Read the model definition and answer for the solid it produces. Units are mm, in the model's axes. Coordinates: 2 decimals unless noted, no trailing zeros. Loops run counter-clockwise (first coordinate to the right, second up) from the corner with the lowest first, then second, coordinate; pieces in that order, holes last. Notation, with made-up numbers: (83, 8) -> (95, 8) arc R14 cw to (95, 12) -> close; hole circle Ø7 at (33, -29.5). An arc over 180 degrees is marked (long way). Answer as a JSON object with one key per item and string values. Group by question number.
Q1. The part is cut by section D-D on x = 9.63. Write down the section's boundary in (y, z) (3 decimals), and give its area (3 significant figures).
Q2. The part is cut by section A-A on x = -12.5. Write down the section's boundary in (y, z) (3 decimals), and give its area (3 significant figures).
Q3. Straight lines are drawn through the part: line 1 along X through (y, z) = (0.7, 9.5); line 2 along X through (y, z) = (0.5, 8.5); line 3 along X through (y, z) = (1.45, -0.5). For each, find the intervals that lie inside material, in ascending order. Write a range as [from, to].
Q4. This flat-tipped pin is pushed along its axis until it touches: P1, Ø1.9, axis at x = 12.5, z = -9.5, coming from the +Y side. Where does it stop, or does it pass through?
Q5. The part is cut by section C-C on z = 9.5. Write down the section's boundary in (x, y) (3 decimals), and give its area (3 significant figures).
Q6. Determine the mould class of faces 1 (the cylindrical face through (13.58, 1.57, -10.68)), 2 (the cylindrical face through (-14.985, 1.61, -11.699)), 3 (the cylindrical face through (14.969, 1.61, 11.715)), 4 (the flat face through (15.27, 2, 0)) for opening direction Z: released by +Z, released by -Z, zero draft, split by the parting line, or undercut.
Q7. The part is cut by section B-B on z = 0. Write down the section's boundary in (x, y) (3 decimals).
from build123d import *

# Parameters (mm, degrees)
SKETCH1_W           = 30.54
SKETCH1_H           = 24
SKETCH1_R           = 1.6
BOSS_EXTRUDE1_DEPTH = 3.175
FILLET1_R           = 1
CUT_EXTRUDE1_REACH  = 21.679
SKETCH3_R           = 1.65


with BuildPart() as part:
    # Sketch1 → Boss-Extrude1 (new body)
    with BuildSketch(Plane(origin=(0, 0, 0), x_dir=(1, 0, 0), z_dir=(0, 1, 0))):
        Rectangle(SKETCH1_W, SKETCH1_H)
        with Locations(Location((-12.5, 9.5, 0), (0, 0, 270))):
            Circle(SKETCH1_R, mode=Mode.SUBTRACT)
        with Locations(Location((-12.5, -9.5, 0), (0, 0, 270))):
            Circle(SKETCH1_R, mode=Mode.SUBTRACT)
        with Locations(Location((12.5, -9.5, 0), (0, 0, 270))):
            Circle(SKETCH1_R, mode=Mode.SUBTRACT)
        with Locations(Location((12.5, 9.5, 0), (0, 0, 270))):
            Circle(SKETCH1_R, mode=Mode.SUBTRACT)
    extrude(amount=BOSS_EXTRUDE1_DEPTH)

    # Fillet1
    fillet1_edges = [part.edges().sort_by_distance(p)[0] for p in [
        (15.27, 1.5875, 12),
        (-15.27, 1.5875, 12),
        (-15.27, 1.5875, -12),
        (15.27, 1.5875, -12),
    ]]
    fillet(fillet1_edges, radius=FILLET1_R)

    # Sketch3 → Cut-Extrude1 (cut, up to next)
    with BuildSketch(Plane(origin=(0, 3.175, 0), x_dir=(1, 0, 0), z_dir=(0, 1, 0)), mode=Mode.PRIVATE) as cut_extrude1_sk1:
        with Locations(Location((9.63, 0, 0), (0, 0, 270))):
            Circle(SKETCH3_R)
    cut_extrude1_tool1 = extrude(cut_extrude1_sk1.sketch, amount=-CUT_EXTRUDE1_REACH, mode=Mode.PRIVATE) & part.part
    add(cut_extrude1_tool1.solids().sort_by_distance((9.63, 3.175, 0))[0], mode=Mode.SUBTRACT)


solid = part.part
Final values:
{
 "1": {"outline": "(0, -12) -> (3.175, -12) -> (3.175, -1.65) -> (0, -1.65) -> close; (0, 1.65) -> (3.175, 1.65) -> (3.175, 12) -> (0, 12) -> close", "area": "65.7 mm2"},
 "2": {"outline": "(0, -12) -> (3.175, -12) -> (3.175, -11.1) -> (0, -11.1) -> close; (0, -7.9) -> (3.175, -7.9) -> (3.175, 7.9) -> (0, 7.9) -> close; (0, 11.1) -> (3.175, 11.1) -> (3.175, 12) -> (0, 12) -> close", "area": "55.9 mm2"},
 "3": {"line 1": "x = [-15.27, -14.1], [-10.9, 10.9], [14.1, 15.27]", "line 2": "x = [-15.27, -13.75], [-11.25, 11.25], [13.75, 15.27]", "line 3": "x = [-15.27, 8.06], [11.2, 15.27]"},
 "4": {"P1": "passes through"},
 "5": {"outline": "(-15.27, 0) -> (-14.1, 0) -> (-14.1, 3.175) -> (-15.27, 3.175) -> close; (-10.9, 0) -> (10.9, 0) -> (10.9, 3.175) -> (-10.9, 3.175) -> close; (14.1, 0) -> (15.27, 0) -> (15.27, 3.175) -> (14.1, 3.175) -> close", "area": "76.6 mm2"},
 "6": {"face 1": "undercut", "face 2": "released by -Z", "face 3": "released by +Z", "face 4": "zero draft"},
 "7": {"outline": "(-15.27, 0) -> (7.98, 0) -> (7.98, 3.175) -> (-15.27, 3.175) -> close; (11.28, 0) -> (15.27, 0) -> (15.27, 3.175) -> (11.28, 3.175) -> close"}
}
